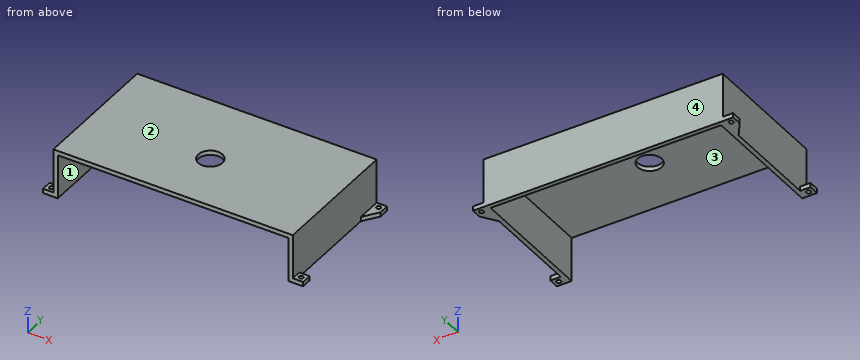
from build123d import *

# Parameters (mm, degrees)
BOSS_EXTRUDE1_DEPTH = 33
SKETCH1_4_R         = 1.5
SKETCH1_4_W         = 7
SKETCH1_4_H         = 7
BOSS_EXTRUDE2_DEPTH = 3
SKETCH3_W           = 156
SKETCH3_H           = 87
SKETCH3_R           = 8.137703122
CUT_EXTRUDE1_DEPTH  = 30
SKETCH3_2_R         = 8.137703122
CUT_EXTRUDE2_DEPTH  = 33


with BuildPart() as part:
    # Sketch1 → Boss-Extrude1 (new body)
    with BuildSketch(Plane.XY):
        Polygon((0, 7), (0, 0), (162, 0), (162, 7), (162, 73), (162, 83), (162, 90), (0, 90), (0, 83), (0, 73), align=None)
    extrude(amount=BOSS_EXTRUDE1_DEPTH)

    # Sketch1_4 → Boss-Extrude2 (add)
    # profile 1 of 6: a face of its own
    with BuildSketch(Plane.XY):
        Polygon((-7, 83), (0, 73), (0, 83), (0, 90), (-7, 90), align=None)
        with Locations((-3.5, 86.5)):
            Circle(SKETCH1_4_R, mode=Mode.SUBTRACT)
    # profile 2 of 6: a face of its own
    with BuildSketch(Plane.XY):
        Polygon((-7, 83), (0, 73), (0, 83), (0, 90), (-7, 90), align=None)
        with Locations((-3.5, 86.5)):
            Circle(SKETCH1_4_R, mode=Mode.SUBTRACT)
    # profile 3 of 6: a face of its own
    with BuildSketch(Plane.XY):
        with Locations((-3.5, 3.5)):
            Rectangle(SKETCH1_4_W, SKETCH1_4_H)
        with Locations((-3.5, 3.5)):
            Circle(SKETCH1_4_R, mode=Mode.SUBTRACT)
    # profile 4 of 6: a face of its own
    with BuildSketch(Plane.XY):
        with Locations((165.5, 3.5)):
            Rectangle(SKETCH1_4_W, SKETCH1_4_H)
        with Locations((165.5, 3.5)):
            Circle(SKETCH1_4_R, mode=Mode.SUBTRACT)
    # profile 5 of 6: a face of its own
    with BuildSketch(Plane.XY):
        Polygon((162, 83), (162, 73), (169, 83), (169, 90), (162, 90), align=None)
        with Locations((165.5, 86.5)):
            Circle(SKETCH1_4_R, mode=Mode.SUBTRACT)
    # profile 6 of 6: a face of its own
    with BuildSketch(Plane.XY):
        Polygon((162, 83), (162, 73), (169, 83), (169, 90), (162, 90), align=None)
        with Locations((165.5, 86.5)):
            Circle(SKETCH1_4_R, mode=Mode.SUBTRACT)
    extrude(amount=BOSS_EXTRUDE2_DEPTH)

    # Sketch3 → Cut-Extrude1 (cut)
    with BuildSketch(Plane(origin=(0, 0, 0), x_dir=(-1, 0, 0), z_dir=(0, 0, -1))):
        with Locations((-81, 43.5)):
            Rectangle(SKETCH3_W, SKETCH3_H)
        with Locations((-81, 40)):
            Circle(SKETCH3_R, mode=Mode.SUBTRACT)
    extrude(amount=-CUT_EXTRUDE1_DEPTH, mode=Mode.SUBTRACT)

    # Sketch3_2 → Cut-Extrude2 (cut)
    with BuildSketch(Plane(origin=(0, 0, 0), x_dir=(-1, 0, 0), z_dir=(0, 0, -1))):
        with Locations((-81, 40)):
            Circle(SKETCH3_2_R)
    extrude(amount=-CUT_EXTRUDE2_DEPTH, mode=Mode.SUBTRACT)


solid = part.part
Input: part model. Units: mm. Frame: model coordinates. Face numbers are marked on the shaded views. A direction names the side the tool comes from. Give positions to 0.01 mm unless a question says otherwise; leave off trailing zeros. Order: outer loops, then holes, each group sorted by start corner. A loop starts at its lowest first (then second) coordinate and runs counter-clockwise, first axis right, second up.
Q1. Contact query for flat-ended pins moving along their axis: pin 1 Ø5 at (x, y) = (101.5, 77) entering from -Z; pin 2 Ø8 at (y, z) = (67.5, 26.5) entering from -X; pin 3 Ø5.5 at (x, y) = (167, 82) entering from +Z. Output: stop coordinate, or through.
Checked values:
pin 1: stops at z = 30
pin 2: stops at x = 0
pin 3: stops at z = 3
Q2. Section B-B on y = 40. Output: boundary loops of the cut face in (x, z).
Checked values:
outline: (0, 0) - (3, 0) - (3, 30) - (72.86, 30) - (72.86, 33) - (0, 33) - close; (89.14, 30) - (159, 30) - (159, 0) - (162, 0) - (162, 33) - (89.14, 33) - close
Q3. Section A-A on x = 81. Output: boundary loops of the cut face in (y, z).
Checked values:
outline: (0, 30) - (31.86, 30) - (31.86, 33) - (0, 33) - close; (48.14, 30) - (87, 30) - (87, 0) - (90, 0) - (90, 33) - (48.14, 33) - close
Q4. Set-up query: the marked faces 1 and 2. Return all of +Z, -Z, +X, -X, +Y, -Y with unobstructed straight access to the full face (end or side cutting, diameter ignored); none if empty.
Checked values:
face 1: -Z, -Y
face 2: +Z, +X, -X, +Y, -Y
Q5. Draft query along X for the marked faces 3 and 4. Return one class per face: +X half, -X half, draft (parallel to the pull), parting line (faces both ways), or undercut.
Checked values:
face 3: undercut
face 4: draft
Q6. Ray query, probe 1 along X at (y, z) = (86.5, 0.75); probe 2 along Y at (x, z) = (165, 2); probe 3 along X at (y, z) = (3, 1). Return the intervals inside material, ascending.
Checked values:
probe 1: x = -7 to -5, -2 to 3, 159 to 164, 167 to 169
probe 2: y = 0 to 2.09, 4.91 to 7, 77.29 to 85.09, 87.91 to 90
probe 3: x = -7 to -4.91, -2.09 to 3, 159 to 164.09, 166.91 to 169
Q7. Section D-D on z = 22.5. Output: boundary loops of the cut face in (x, y), and give its area (3 significant figures).
Checked values:
outline: (0, 0) - (3, 0) - (3, 87) - (159, 87) - (159, 0) - (162, 0) - (162, 90) - (0, 90) - close
area: 1,010 mm2
Q8. Section C-C on y = 62. Output: boundary loops of the cut face in (x, z), and give its area (3 significant figures).
Checked values:
outline: (0, 0) - (3, 0) - (3, 30) - (159, 30) - (159, 0) - (162, 0) - (162, 33) - (0, 33) - close
area: 666 mm2
